Verification items for the finished model (mm, model axes). Face numbers are marked on the shaded views. A direction names the side the tool comes from. Coordinates: 2 decimals unless noted, no trailing zeros. Loops run counter-clockwise (first coordinate to the right, second up) from the corner with the lowest first, then second, coordinate; pieces in that order, holes last. Notation, with made-up numbers: (18, -17.75) -> (41, -17.75) arc R23 ccw to (41, -4.75) -> close; hole circle Ø9 at (56, 64.25). An arc over 180 degrees is marked (long way). Write item = value, one per line.
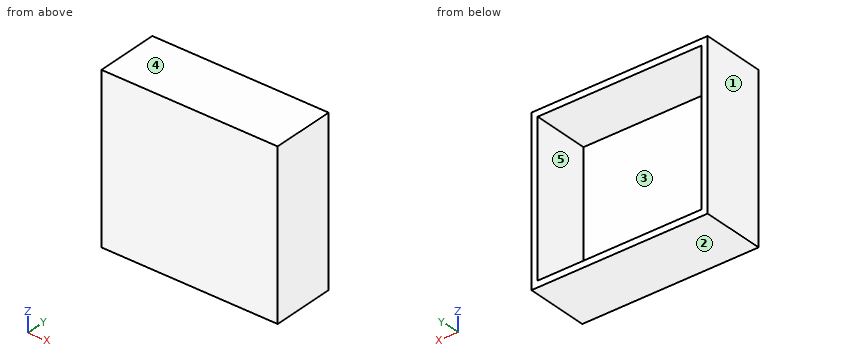
```python
from build123d import *

# Parameters (mm, degrees)
SKETCH_1_W          = 140
SKETCH_1_H          = 130
EXTRUDE_2_DEPTH     = 25
SKETCH_4_W          = 130
SKETCH_4_H          = 120
CUT_EXTRUDE_1_DEPTH = 45


with BuildPart() as part:
    # 草圖1 → 填料-伸長2 (new, symmetric)
    with BuildSketch(Plane(origin=(0, 0, 0), x_dir=(1, 0, 0), z_dir=(0, 1, 0))):
        Rectangle(SKETCH_1_W, SKETCH_1_H)
    extrude(amount=EXTRUDE_2_DEPTH, both=True)

    # 草圖4 → 除料-伸長1 (cut)
    with BuildSketch(Plane(origin=(0, 25, 0), x_dir=(1, 0, 0), z_dir=(0, 1, 0))):
        Rectangle(SKETCH_4_W, SKETCH_4_H)
    extrude(amount=-CUT_EXTRUDE_1_DEPTH, mode=Mode.SUBTRACT)


solid = part.part
```
1) Release check for a two-part mould opening along Z. For the marked faces 1, 2 and 3 record: pulls with the +Z half, pulls with the -Z half, needs draft (parallel to the pull), parting line crosses it, or undercut.
Ans:
face_1 = needs draft
face_2 = pulls with the -Z half
face_3 = undercut
2) Tool access check on the marked faces 4 and 5. Record the directions out of +Z, -Z, +X, -X, +Y, -Y that give a thin tool (end or side, any length) a straight path to the whole face; none if there is none.
Ans:
face_4 = +Z, +X, -X, +Y, -Y
face_5 = +Y
3) Sectioned sample at B-B, the plane z = -7. Record the cut outline in (x, y).
Ans:
outline = (-70, -25) -> (70, -25) -> (70, 25) -> (65, 25) -> (65, -20) -> (-65, -20) -> (-65, 25) -> (-70, 25) -> close
4) Sectioned sample at A-A, the plane y = -16. Record the cut outline in (x, z), plus the area to 3 significant figures.
Ans:
outline = (-70, -65) -> (70, -65) -> (70, 65) -> (-70, 65) -> close; hole (-65, -60) -> (65, -60) -> (65, 60) -> (-65, 60) -> close
area = 2,600 mm2
5) Sectioned sample at C-C, the plane x = 50. Record the cut outline in (y, z).
Ans:
outline = (-25, -65) -> (25, -65) -> (25, -60) -> (-20, -60) -> (-20, 60) -> (25, 60) -> (25, 65) -> (-25, 65) -> close
6) Material ranges on line 1 (X direction, y = 19.5, z = -20); line 2 (Z direction, x = -19.5, y = -15); line 3 (Y direction, x = -12.5, z = -41.5), recorded low to high.
Ans:
line_1 = -70 to -65, 65 to 70
line_2 = -65 to -60, 60 to 65
line_3 = -25 to -20
7) Depth check by flat-ended pin: pin 1 Ø4 at (x, z) = (-8.5, -16.5) entering from +Y. Enter the tip coordinate at first touch or a pass-through.
Ans:
pin_1 = -20
